Here's how the part is built. I have some questions about the finished solid (model axes, mm). Coordinates: 2 decimals unless noted, no trailing zeros. Loops run counter-clockwise (first coordinate to the right, second up) from the corner with the lowest first, then second, coordinate; pieces in that order, holes last. Notation, with made-up numbers: (67.5, 49.5) -> (111.5, 49.5) arc R28 cw to (111.5, 82.5) -> close; hole circle Ø11 at (35.5, -31). An arc over 180 degrees is marked (long way). Answer as a JSON object with one key per item and string values. Group by question number.
Q1. I want a section at A-A on x = -16. Write out the boundary of the cut face in (y, z).
Q2. I need wall thicknesses on line 1 (Y direction, x = 0, z = 0.4); line 2 (Y direction, x = -16, z = 0.4); line 3 (X direction, y = -2.25, z = 0.35). Which ranges of each line are inside material? Lowest first, please.
Q3. Thinking about a two-plate mould opening in X: for faces 1 (the cylindrical face through (-9.6, -1.2, 0.5)), 2 (the flat face through (-4, 0, 0)), 3 (the flat face through (14, -0.1, 0.5)), which applies, released by +X, released by -X, zero draft, split by the parting line, or undercut?
Q4. I want a section at C-C on x = -8. Write out the boundary of the cut face in (y, z), then the cut area to 3 significant figures.
Q5. I'm going to push a flat-ended pin straight in: pin 1 (3 mm diameter, centred on x = -16, y = 0, fed in from +Z). Where does the tip first touch, or does it pass through?
Q6. I want a section at B-B on z = 0.5. Write out the boundary of the cut face in (x, y).
```python
from build123d import *

# Parameters (mm, degrees)
F0_W     = 36
F0_H     = 8
F0_R     = 2.5
F0_R_2   = 2
F0_R_3   = 1.5
F0_R_4   = 1
F0_R_5   = 0.5
F1_DEPTH = 1


with BuildPart() as f1:
    # F0 (on Top) → F1 (new body)
    with BuildSketch(Plane.XY):
        with Locations((-4, 0)):
            Rectangle(F0_W, F0_H)
        with Locations((-16, 0)):
            Circle(F0_R, mode=Mode.SUBTRACT)
        with Locations((-8, 0)):
            Circle(F0_R_2, mode=Mode.SUBTRACT)
        Circle(F0_R_3, mode=Mode.SUBTRACT)
        with Locations((6, 0)):
            Circle(F0_R_4, mode=Mode.SUBTRACT)
        with Locations((10, 0)):
            Circle(F0_R_5, mode=Mode.SUBTRACT)
    extrude(amount=F1_DEPTH)


solid = f1.part
```
Result set:
{
 "1": {"outline": "(-4, 0) -> (-2.5, 0) -> (-2.5, 1) -> (-4, 1) -> close; (2.5, 0) -> (4, 0) -> (4, 1) -> (2.5, 1) -> close"},
 "2": {"line 1": "y = -4 to -1.5, 1.5 to 4", "line 2": "y = -4 to -2.5, 2.5 to 4", "line 3": "x = -22 to -17.09, -14.91 to 14"},
 "3": {"face 1": "undercut", "face 2": "zero draft", "face 3": "released by +X"},
 "4": {"outline": "(-4, 0) -> (-2, 0) -> (-2, 1) -> (-4, 1) -> close; (2, 0) -> (4, 0) -> (4, 1) -> (2, 1) -> close", "area": "4.00 mm²"},
 "5": {"pin 1": "passes through"},
 "6": {"outline": "(-22, -4) -> (14, -4) -> (14, 4) -> (-22, 4) -> close; hole circle Ø5 at (-16, 0); hole circle Ø4 at (-8, 0); hole circle Ø3 at (0, 0); hole circle Ø2 at (6, 0); hole circle Ø1 at (10, 0)"}
}
